Work out the finished part from the listing and answer in its coordinate system (mm). Round coordinates to 2 decimals unless told otherwise and drop trailing zeros. Loops run counter-clockwise (first coordinate to the right, second up) from the corner with the lowest first, then second, coordinate; pieces in that order, holes last.
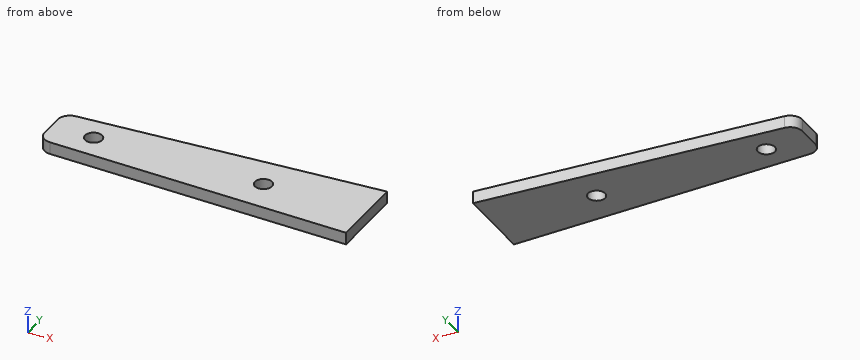
from build123d import *

# Parameters (mm, degrees)
BOSS_EXTRUDE1_DEPTH  = 3.175
M4_CLEARANCE_HOLE2_D = 4.5
FILLET1_R            = 3.175


with BuildPart() as part:
    # Sketch1 → Boss-Extrude1 (new body)
    with BuildSketch(Plane.XY):
        Polygon((49.2125, 10.280952381), (-33.3375, 6.35), (-33.3375, -6.35), (49.2125, -10.280952381), align=None)
    extrude(amount=BOSS_EXTRUDE1_DEPTH)

    # M4 Clearance Hole2 (through all)
    with Locations(Plane.XY.offset(3.175)):
        with Locations((-22.225, 0), (22.225, 0)):
            Hole(M4_CLEARANCE_HOLE2_D / 2)

    # Fillet1
    fillet1_edges = [part.edges().sort_by_distance(p)[0] for p in [
        (-33.3375, -6.35, 1.5875),
        (-33.3375, 6.35, 1.5875),
    ]]
    fillet(fillet1_edges, radius=FILLET1_R)


solid = part.part
Item 1: Section D-D, the plane y = 8 is taken. Give the vertices of the cut face in (x, z) (1 decimal), plus the area to 3 significant figures.
Item 2: Straight lines are drawn through the part: line 1 (X direction, y = -0.25, z = 2.5); line 2 (X direction, y = 1.75, z = 2.4); line 3 (Y direction, x = 20.5, z = 1.9). For each, find the intervals that lie inside material, in ascending order.
Item 3: Section C-C, the plane x = -14.5 is taken. Give the vertices of the cut face in (y, z) (3 decimals).
Item 4: Section B-B, the plane z = 0.95 is taken. State how many separate pieces and enclosed holes the cut face has, plus the area to 3 significant figures.
Item 5: Section A-A, the plane y = 0 is taken. Give the vertices of the cut face in (x, z) (1 decimal), plus the area to 3 significant figures.
Answer below:
1. outline: (1.3, 0) - (49.2, 0) - (49.2, 3.2) - (1.3, 3.2) - close
1. area: 152 mm2
2. line 1: x = -33.34 to -24.46, -19.99 to 19.99, 24.46 to 49.21
2. line 2: x = -33.34 to -23.64, -20.81 to 20.81, 23.64 to 49.21
2. line 3: y = -8.91 to -1.44, 1.44 to 8.91
3. outline: (-7.247, 0) - (7.247, 0) - (7.247, 3.175) - (-7.247, 3.175) - close
4. separate pieces: 1
4. enclosed holes: 2
4. area: 1,340 mm2
5. outline: (-33.3, 0) - (-24.5, 0) - (-24.5, 3.2) - (-33.3, 3.2) - close; (-20, 0) - (20, 0) - (20, 3.2) - (-20, 3.2) - close; (24.5, 0) - (49.2, 0) - (49.2, 3.2) - (24.5, 3.2) - close
5. area: 234 mm2
